from build123d import *

# Parameters (mm, degrees)
SKETCH1_R                  = 6.4
BOSS_EXTRUDE1_DEPTH        = 152.53
F_10_24_TAPPED_HOLE1_D     = 3.7973
F_10_24_TAPPED_HOLE1_DEPTH = 12.83
F_10_24_TAPPED_HOLE1_TIP   = 1.140824014
F_10_24_TAPPED_HOLE2_D     = 3.7973
F_10_24_TAPPED_HOLE2_DEPTH = 12.83
F_10_24_TAPPED_HOLE2_TIP   = 1.140824014


with BuildPart() as part:
    # Sketch1 → Boss-Extrude1 (new body)
    with BuildSketch(Plane.XY):
        Circle(SKETCH1_R)
    extrude(amount=BOSS_EXTRUDE1_DEPTH)

    # #10-24 Tapped Hole1
    with Locations(Plane(origin=(0, 0, 0), x_dir=(-1, 0, 0), z_dir=(0, 0, -1))):
        with Locations((0, 0)):
            Hole(F_10_24_TAPPED_HOLE1_D / 2, depth=F_10_24_TAPPED_HOLE1_DEPTH)
            with Locations((0, 0, -(F_10_24_TAPPED_HOLE1_DEPTH + F_10_24_TAPPED_HOLE1_TIP / 2))):  # 118° drill point
                Cone(0, F_10_24_TAPPED_HOLE1_D / 2, F_10_24_TAPPED_HOLE1_TIP, mode=Mode.SUBTRACT)

    # #10-24 Tapped Hole2
    with Locations(Plane.XY.offset(152.53)):
        with Locations((0, 0)):
            Hole(F_10_24_TAPPED_HOLE2_D / 2, depth=F_10_24_TAPPED_HOLE2_DEPTH)
            with Locations((0, 0, -(F_10_24_TAPPED_HOLE2_DEPTH + F_10_24_TAPPED_HOLE2_TIP / 2))):  # 118° drill point
                Cone(0, F_10_24_TAPPED_HOLE2_D / 2, F_10_24_TAPPED_HOLE2_TIP, mode=Mode.SUBTRACT)


solid = part.part
Here's how the part is built. I have some questions about the finished solid (model axes, mm). A direction names the side the tool comes from. Coordinates: 2 decimals unless noted, no trailing zeros. Order: outer loops, then holes, each group sorted by start corner. A loop starts at its lowest first (then second) coordinate and runs counter-clockwise, first axis right, second up. Notation, with made-up numbers: M -18,-31.5 L 21,-31.5 A20 ccw 21,-13.5 Z; hole C 33.25,24.25 d8. An arc over 180 degrees is marked long. Answer as CSV lines item,"result". Start each with the question number.
1. For pin 1 (1.5 mm diameter, centred on x = -4.5, z = 66.5, fed in from +Y); pin 2 (3.5 mm diameter, centred on x = 0, y = 0, fed in from -Z); pin 3 (4 mm diameter, centred on x = -4, z = 51, fed in from -Y), each with a flat end and sliding along its axis, tell me the tip position at first contact or that it passes through.
2. I want a section at A-A, the plane z = 113.5. Write out the boundary of the cut face in (x, y), and give its area (3 significant figures).
3. I want a section at B-B, the plane x = -5. Write out the boundary of the cut face in (y, z) (3 decimals).
4. We'd pull the mould along Y, two halves only. Please class faces 1 (the cylindrical face through (-5.08, -3.89, 75.2)), 2 (the conical face through (-0.18, 0.28, 13.77)), 3 (the flat face through (1, 2, 152.53)): released by +Y, released by -Y, zero draft, split by the parting line, or undercut.
5. I need wall thicknesses on line 1 (Y direction, x = 0, z = 146); line 2 (Y direction, x = 2.5, z = 58); line 3 (X direction, y = -5.25, z = 48.5). Which ranges of each line are inside material? Lowest first, please. Write a range as [from, to].
6. I want a section at C-C, the plane y = -3.5. Write out the boundary of the cut face in (x, z), and give its area (3 significant figures).
7. On a 3-axis mill with a long thin cutter (end or side, diameter ignored), from which of +Z, -Z, +X, -X, +Y, -Y can I reach the whole of each face in a straight line? I mean faces 4 (the flat face through (1, 2, 0)), 5 (the cylindrical face through (-1.8, 0.6, 146)), 6 (the cylindrical face through (1.8, 0.6, 6.5)). Say none if no direction works.
Recorded:
1,pin 1,"stops at y = 5.19"
1,pin 2,"stops at z = 12.92"
1,pin 3,"stops at y = -6.08"
2,outline,"C 0,0 d12.8"
2,area,"129 mm2"
3,outline,"M -3.995,0 L 3.995,0 L 3.995,152.53 L -3.995,152.53 Z"
4,face 1,"split by the parting line"
4,face 2,"undercut"
4,face 3,"zero draft"
5,line 1,"y = [-6.4, -1.9], [1.9, 6.4]"
5,line 2,"y = [-5.89, 5.89]"
5,line 3,"x = [-3.66, 3.66]"
6,outline,"M -5.36,0 L 5.36,0 L 5.36,152.53 L -5.36,152.53 Z"
6,area,"1,630 mm2"
7,face 4,"-Z, +X, -X, +Y, -Y"
7,face 5,"+Z"
7,face 6,"-Z"
